The listing builds one solid part. Answer for the finished solid, in the listing's coordinates (mm). A direction names the side the tool comes from. Round coordinates to 2 decimals unless told otherwise and drop trailing zeros. Loops run counter-clockwise (first coordinate to the right, second up) from the corner with the lowest first, then second, coordinate; pieces in that order, holes last. Notation, with made-up numbers: (40, 83) - (85, 83) arc R17 ccw to (85, 89) - close; hole circle Ø4 at (81, 6). An arc over 180 degrees is marked (long way). One line per question, with ' | ' between items. Start each with the question number.
Autodesk Inventor part; units mm, degrees
ref_plane "YZ Plane" through (0, 0, 0) normal (1, 0, 0) x (0, 1, 0)
ref_plane "XZ Plane" through (0, 0, 0) normal (0, 1, 0) x (-1, 0, 0)
ref_plane "XY Plane" through (0, 0, 0) normal (0, 0, 1) x (1, 0, 0)
sketch "Sketch1" plane through (0, 0, 0) normal (0, 0, 1) x (1, 0, 0)
  line L0 (-63, 30) -> (63, 30)
  line L1 (63, 30) -> (63, -30)
  line L2 (63, -30) -> (-63, -30)
  line L3 (-63, -30) -> (-63, 30)
  line L4 (-63, 30) -> (63, -30) construction
  line L5 (63, 30) -> (-63, -30) construction
  line L6 (-63, 30) -> (63, 30) construction
  point P0 (0, 0)
  dimension "d0" = 126
  dimension "d1" = 0
  dimension "d2" = 60
extrude "Extrusion1" add sketch "Sketch1" along normal blind 10
sketch "Sketch2" plane through (-63, -30, 0) normal (-1, 0, 0) x (0, 0, 1)
  line L0 (0, 60) -> (10, 60)
  line L1 (5, 60) -> (5, 49)
  circle A0 centre (5, 49) radius 2
  point P0 (0, 30)
  dimension "d5" = 11
  dimension "d6" = 4
extrude "Extrusion2" cut sketch "Sketch2" against normal blind 5.5
pattern_linear "Rectangular Pattern1" count 2 spacing 120.5 along (1, 0, 0) count 2 spacing -38 along (0, 1, 0) of "Extrusion2"
ref_plane "Work Plane1" through (-63, 0, 0) normal (0, 1, 0) x (1, 0, 0)
sketch "Sketch3" plane through (-63, -30, 0) normal (0, -1, 0) x (1, 0, 0)
  line L0 (0, 0) -> (0, 10)
  line L1 (126, 0) -> (0, 0)
  line L2 (0, 10) -> (126, 10)
  line L3 (126, 10) -> (126, 0)
  line L4 (126, 0) -> (0, 0)
  line L5 (0, 0) -> (0, 10)
  point P0 (63, 0)
extrude "Extrusion3" add sketch "Sketch3" along normal blind 1
mirror "Mirror1" about plane through (-63, 0, 0) normal (0, 1, 0) of "Extrusion3"
properties part number "basetemplate"
(1) Consider L1, parallel to Y at x = -59.05, z = 5; L2, parallel to Z at x = -61.05, y = 19; L3, parallel to X at y = -19, z = 6.5. Determine where each line is inside the solid, lowest interval first.
(2) A tool of negligible diameter and unlimited length cuts with its end or side. For faces 1 (the cylindrical face through (-60, -17, 5)), 2 (the flat face through (63, 0, 5)), 3 (the cylindrical face through (60, 21, 5)), from which of +Z, -Z, +X, -X, +Y, -Y can it reach the whole face along a straight path? Write none if from no direction.
(3) Find section A-A on y = 19. Write down the section's boundary in (x, z).
(4) Determine the mould class of faces 4 (the flat face through (-1, 0, 0)), 5 (the flat face through (57.5, -19, 5)), 6 (the flat face through (-1, -31, 5)) for opening direction Z: pulls with the +Z half, pulls with the -Z half, needs draft (parallel to the pull), parting line crosses it, or undercut.
(5) This flat-tipped pin is pushed along its axis until it touches: P1, Ø2.5, axis at y = -19, z = 5, coming from the -X side. Where does it stop, or does it pass through?
Answer below:
1) L1: -31 to -21, -17 to 17, 21 to 31 | L2: 0 to 3, 7 to 10 | L3: -57.5 to 57.5
2) face 1: -X | face 2: +Z, -Z, +X, +Y, -Y | face 3: +X
3) outline: (-63, 0) - (63, 0) - (63, 3) - (57.5, 3) - (57.5, 7) - (63, 7) - (63, 10) - (-63, 10) - (-63, 7) - (-57.5, 7) - (-57.5, 3) - (-63, 3) - close
4) face 4: pulls with the -Z half | face 5: undercut | face 6: needs draft
5) P1: x = -57.5
